Input: part model. Units: mm. Frame: model coordinates. A direction names the side the tool comes from. Round coordinates to 2 decimals unless told otherwise and drop trailing zeros. Write each loop counter-clockwise with the first axis right and the second up, starting at its lowest first coordinate (ties: lowest second). Pieces come first, ordered by that corner, then holes. Notation, with made-up numbers: (27.25, 60) -> (81.25, 60) arc R30 ccw to (81.25, 91) -> close; hole circle Ø2 at (0, 65.5). An arc over 180 degrees is marked (long way). Write item = value, one per line.
```python
from build123d import *

# Parameters (mm, degrees)
SKETCH1_W           = 127
SKETCH1_H           = 76.2
BOSS_EXTRUDE1_DEPTH = 2
BOSS_EXTRUDE2_DEPTH = 203.2
FILLET2_R           = 25
FILLET3_R           = 15
FILLET4_R           = 1


with BuildPart() as part:
    # Sketch1 → Boss-Extrude1 (new body)
    with BuildSketch(Plane(origin=(0, 0, 0), x_dir=(1, 0, 0), z_dir=(0, 1, 0))):
        with Locations((32.767173068, 3.871122995)):
            Rectangle(SKETCH1_W, SKETCH1_H)
        Polygon((96.267173068, -34.228877005), (98.330615884, -36.163354646), (-32.796269749, -36.163354646), (-32.796269749, 43.905600635), (-30.732826932, 41.971122995), (-30.732826932, -34.228877005), align=None)
        Polygon((96.267173068, 41.971122995), (96.267173068, -34.228877005), (98.330615884, -36.163354646), (98.330615884, 43.905600635), align=None)
        Polygon((-30.732826932, 41.971122995), (96.267173068, 41.971122995), (98.330615884, 43.905600635), (-32.796269749, 43.905600635), align=None)
    extrude(amount=BOSS_EXTRUDE1_DEPTH)

    # Sketch1<3> → Boss-Extrude2 (add)
    with BuildSketch(Plane(origin=(0, 0, 0), x_dir=(1, 0, 0), z_dir=(0, 1, 0))):
        Polygon((96.267173068, 41.971122995), (96.267173068, -34.228877005), (98.330615884, -36.163354646), (98.330615884, 43.905600635), align=None)
        Polygon((-30.732826932, 41.971122995), (96.267173068, 41.971122995), (98.330615884, 43.905600635), (-32.796269749, 43.905600635), align=None)
        Polygon((96.267173068, -34.228877005), (98.330615884, -36.163354646), (-32.796269749, -36.163354646), (-32.796269749, 43.905600635), (-30.732826932, 41.971122995), (-30.732826932, -34.228877005), align=None)
    extrude(amount=BOSS_EXTRUDE2_DEPTH)

    # Fillet2
    fillet2_edges = [part.edges().sort_by_distance(p)[0] for p in [
        (96.267173068, 102.6, -41.971122995),
        (96.267173068, 102.6, 34.228877005),
        (-30.732826932, 102.6, 34.228877005),
        (-30.732826932, 102.6, -41.971122995),
        (98.330615884, 101.6, 36.163354646),
        (-32.796269749, 101.6, 36.163354646),
        (-32.796269749, 101.6, -43.905600635),
        (98.330615884, 101.6, -43.905600635),
    ]]
    fillet(fillet2_edges, radius=FILLET2_R)

    # Fillet3
    fillet3_edges = [part.edges().sort_by_distance(p)[0] for p in [
        (32.767173068, 2, -41.971122995),
        (32.767173068, 2, 34.228877005),
        (96.267173068, 2, -3.871122995),
        (-30.732826932, 2, -3.871122995),
        (88.944842597, 2, -34.648792524),
        (88.944842597, 2, 26.906546535),
        (-23.410496462, 2, 26.906546535),
        (-23.410496462, 2, -34.648792524),
    ]]
    fillet(fillet3_edges, radius=FILLET3_R)

    # Fillet4
    # the kernel refuses this fillet: 1 mm, written as the material it takes off along each edge
    with BuildSketch(Plane(origin=(-32.796269749, 203.2, 11.163354646), x_dir=(1, 0, 0), z_dir=(0, 0, -1))) as fillet4_piece_1:
        with BuildLine():
            CenterArc((FILLET4_R, FILLET4_R), FILLET4_R, 180, 90)
            Line((0, FILLET4_R), (0, 0))
            Line((0, 0), (FILLET4_R, 0))
        make_face()
    extrude(amount=30.068955281, mode=Mode.SUBTRACT)
    with BuildSketch(Plane(origin=(73.330615884, 203.2, -43.905600635), x_dir=(0, 0, 1), z_dir=(-1, 0, 0))) as fillet4_piece_2:
        with BuildLine():
            CenterArc((FILLET4_R, -FILLET4_R), FILLET4_R, 90, 90)
            Line((0, -FILLET4_R), (0, 0))
            Line((0, 0), (FILLET4_R, 0))
        make_face()
    extrude(amount=81.126885633, mode=Mode.SUBTRACT)
    with BuildSketch(Plane(origin=(73.330615884, 203.2, 36.163354646), x_dir=(0, 0, -1), z_dir=(-1, 0, 0))) as fillet4_piece_3:
        with BuildLine():
            CenterArc((FILLET4_R, FILLET4_R), FILLET4_R, 180, 90)
            Line((0, FILLET4_R), (0, 0))
            Line((0, 0), (FILLET4_R, 0))
        make_face()
    extrude(amount=81.126885633, mode=Mode.SUBTRACT)
    with BuildSketch(Plane(origin=(98.330615884, 203.2, 11.163354646), x_dir=(-1, 0, 0), z_dir=(0, 0, -1))) as fillet4_piece_4:
        with BuildLine():
            CenterArc((FILLET4_R, -FILLET4_R), FILLET4_R, 90, 90)
            Line((0, -FILLET4_R), (0, 0))
            Line((0, 0), (FILLET4_R, 0))
        make_face()
    extrude(amount=30.068955281, mode=Mode.SUBTRACT)
    with BuildSketch(Plane(origin=(-5.732826932, 203.2, -41.971122995), x_dir=(0, 0, -1), z_dir=(1, 0, 0))) as fillet4_piece_5:
        with BuildLine():
            CenterArc((FILLET4_R, -FILLET4_R), FILLET4_R, 90, 90)
            Line((0, -FILLET4_R), (0, 0))
            Line((0, 0), (FILLET4_R, 0))
        make_face()
    extrude(amount=77, mode=Mode.SUBTRACT)
    with BuildSketch(Plane(origin=(-30.732826932, 203.2, -16.971122995), x_dir=(-1, 0, 0), z_dir=(0, 0, 1)), Plane(origin=(96.267173068, 203.2, -16.971122995), x_dir=(0, -1, 0), z_dir=(0, 0, 1))) as fillet4_piece_6:
        with BuildLine():
            CenterArc((FILLET4_R, FILLET4_R), FILLET4_R, 180, 90)
            Line((0, FILLET4_R), (0, 0))
            Line((0, 0), (FILLET4_R, 0))
        make_face()
    extrude(amount=26.2, mode=Mode.SUBTRACT)
    with BuildSketch(Plane(origin=(-5.732826932, 203.2, 34.228877005), x_dir=(0, 0, 1), z_dir=(1, 0, 0))) as fillet4_piece_7:
        with BuildLine():
            CenterArc((FILLET4_R, FILLET4_R), FILLET4_R, 180, 90)
            Line((0, FILLET4_R), (0, 0))
            Line((0, 0), (FILLET4_R, 0))
        make_face()
    extrude(amount=77, mode=Mode.SUBTRACT)
    with BuildSketch(Plane(origin=(-5.732826932, 203.2, -16.971122995), x_dir=(0, 0, -1), z_dir=(1, 0, 0))) as fillet4_piece_8:
        with BuildLine():
            CenterArc((25 + FILLET4_R, -FILLET4_R), FILLET4_R, 90, 90)
            Line((25, -FILLET4_R), (25, 0))
            Line((25, 0), (25 + FILLET4_R, 0))
        make_face()
    revolve(axis=Axis((-5.732826932, 203.2, -16.971122995), (0, 1, 0)), revolution_arc=90, mode=Mode.SUBTRACT)
    with BuildSketch(Plane(origin=(-5.732826932, 203.2, 9.228877005), x_dir=(-1, 0, 0), z_dir=(0, 0, -1))) as fillet4_piece_9:
        with BuildLine():
            CenterArc((25 + FILLET4_R, -FILLET4_R), FILLET4_R, 90, 90)
            Line((25, -FILLET4_R), (25, 0))
            Line((25, 0), (25 + FILLET4_R, 0))
        make_face()
    revolve(axis=Axis((-5.732826932, 203.2, 9.228877005), (0, 1, 0)), revolution_arc=90, mode=Mode.SUBTRACT)
    with BuildSketch(Plane(origin=(71.267173068, 203.2, 9.228877005), x_dir=(0, 0, 1), z_dir=(-1, 0, 0))) as fillet4_piece_10:
        with BuildLine():
            CenterArc((25 + FILLET4_R, -FILLET4_R), FILLET4_R, 90, 90)
            Line((25, -FILLET4_R), (25, 0))
            Line((25, 0), (25 + FILLET4_R, 0))
        make_face()
    revolve(axis=Axis((71.267173068, 203.2, 9.228877005), (0, 1, 0)), revolution_arc=90, mode=Mode.SUBTRACT)
    with BuildSketch(Plane(origin=(71.267173068, 203.2, -16.971122995), x_dir=(0, 0, -1), z_dir=(-1, 0, 0))) as fillet4_piece_11:
        with BuildLine():
            CenterArc((25 + FILLET4_R, FILLET4_R), FILLET4_R, 180, 90)
            Line((25 + FILLET4_R, 0), (25, 0))
            Line((25, 0), (25, FILLET4_R))
        make_face()
    revolve(axis=Axis((71.267173068, 203.2, -16.971122995), (0, -1, 0)), revolution_arc=90, mode=Mode.SUBTRACT)
    with BuildSketch(Plane(origin=(73.330615884, 203.2, -18.905600635), x_dir=(1, 0, 0), z_dir=(0, 0, 1))) as fillet4_piece_12:
        with BuildLine():
            CenterArc((25 - FILLET4_R, -FILLET4_R), FILLET4_R, 0, 90)
            Line((25, -FILLET4_R), (25, 0))
            Line((25, 0), (25 - FILLET4_R, 0))
        make_face()
    revolve(axis=Axis((73.330615884, 203.2, -18.905600635), (0, 1, 0)), revolution_arc=90, mode=Mode.SUBTRACT)
    with BuildSketch(Plane(origin=(73.330615884, 203.2, 11.163354646), x_dir=(1, 0, 0), z_dir=(0, 0, -1))) as fillet4_piece_13:
        with BuildLine():
            CenterArc((25 - FILLET4_R, FILLET4_R), FILLET4_R, 270, 90)
            Line((25, FILLET4_R), (25, 0))
            Line((25, 0), (25 - FILLET4_R, 0))
        make_face()
    revolve(axis=Axis((73.330615884, 203.2, 11.163354646), (0, -1, 0)), revolution_arc=90, mode=Mode.SUBTRACT)
    with BuildSketch(Plane(origin=(-7.796269749, 203.2, 11.163354646), x_dir=(-1, 0, 0), z_dir=(0, 0, -1))) as fillet4_piece_14:
        with BuildLine():
            CenterArc((25 - FILLET4_R, -FILLET4_R), FILLET4_R, 0, 90)
            Line((25, -FILLET4_R), (25, 0))
            Line((25, 0), (25 - FILLET4_R, 0))
        make_face()
    revolve(axis=Axis((-7.796269749, 203.2, 11.163354646), (0, 1, 0)), revolution_arc=90, mode=Mode.SUBTRACT)
    with BuildSketch(Plane(origin=(-7.796269749, 203.2, -18.905600635), x_dir=(0, 0, -1), z_dir=(1, 0, 0))) as fillet4_piece_15:
        with BuildLine():
            CenterArc((25 - FILLET4_R, -FILLET4_R), FILLET4_R, 0, 90)
            Line((25, -FILLET4_R), (25, 0))
            Line((25, 0), (25 - FILLET4_R, 0))
        make_face()
    revolve(axis=Axis((-7.796269749, 203.2, -18.905600635), (0, 1, 0)), revolution_arc=90, mode=Mode.SUBTRACT)


solid = part.part
```
1) Cut plane A-A (y = 24). Return the cut outline in (x, z), and give its area (3 significant figures).
Solutions:
outline = (-32.8, -18.91) arc R25 ccw to (-7.8, -43.91) -> (73.33, -43.91) arc R25 ccw to (98.33, -18.91) -> (98.33, 11.16) arc R25 ccw to (73.33, 36.16) -> (-7.8, 36.16) arc R25 ccw to (-32.8, 11.16) -> close; hole (-30.73, -16.97) arc R25 ccw to (-5.73, -41.97) -> (71.27, -41.97) arc R25 ccw to (96.27, -16.97) -> (96.27, 9.23) arc R25 ccw to (71.27, 34.23) -> (-5.73, 34.23) arc R25 ccw to (-30.73, 9.23) -> close
area = 822 mm^2
2) Cut plane C-C (x = 20.5). Return the cut outline in (y, z), and give its area (3 significant figures).
Solutions:
outline = (0, -43.91) -> (202.2, -43.91) arc R1 ccw to (203.2, -42.94) arc R1 ccw to (202.2, -41.97) -> (17, -41.97) arc R15 cw to (2, -26.97) -> (2, 19.23) arc R15 cw to (17, 34.23) -> (202.2, 34.23) arc R1 ccw to (203.2, 35.2) arc R1 ccw to (202.2, 36.16) -> (0, 36.16) -> close
area = 1,030 mm^2
3) Line query: L1, parallel to X at y = 163.5, z = 0; L2, parallel to Z at x = 56, y = 19; L3, parallel to Y at x = 5, z = 15.5. Output: solid intervals per line, ascending. Write a range as from..to.
Solutions:
L1 = -32.8..-30.73, 96.27..98.33
L2 = -43.91..-41.97, 34.23..36.16
L3 = 0..2
4) First-contact query: P1, Ø2, axis at y = 182.5, z = 22.5, coming from the +X side; P2, Ø1, axis at x = 37.5, z = -33, coming from the +Y side; P3, Ø23, axis at x = 16, z = -2, coming from the +Y side. Flat tips, straight axial feed; report the tip coordinate or a pass-through.
Solutions:
P1 = 96.09
P2 = 3.5
P3 = 2
5) Access query for faces 5 (the face through (-26.455, 6.511, -3.688)), 6 (the face through (-25.667, 99.685, -36.388)). Directions: +Z, -Z, +X, -X, +Y, -Y. A direction counts if a zero-diameter tool reaches every point of the face in a straight line with its end or side. Return the directions, or none.
Solutions:
face_5 = +Y
face_6 = -Z, -X, +Y, -Y
6) Draft query along X for faces 1 (the face through (91.2, 99.68, -36.39)), 2 (the face through (-32.796, 100, -4)), 3 (the face through (-23.22, 110.9, -34.84)), 4 (the face through (-23.604, 110.896, 26.711)). Return one class per face: +X half, -X half, draft (parallel to the pull), parting line (faces both ways), or undercut.
Solutions:
face_1 = +X half
face_2 = -X half
face_3 = undercut
face_4 = undercut
7) Cut plane B-B (z = -3.5). Return the cut outline in (x, y), and give its area (3 significant figures).
Solutions:
outline = (-32.8, 0) -> (98.33, 0) -> (98.33, 202.2) arc R1 ccw to (97.33, 203.2) -> (97.27, 203.2) arc R1 ccw to (96.27, 202.2) -> (96.27, 17) arc R15 cw to (81.27, 2) -> (-15.73, 2) arc R15 cw to (-30.73, 17) -> (-30.73, 202.2) arc R1 ccw to (-31.73, 203.2) -> (-31.8, 203.2) arc R1 ccw to (-32.8, 202.2) -> close
area = 1,190 mm^2
